Part print with two shaded views. Sizes in mm from the minimum x, y, z corner. A direction names the side the tool comes from. Round coordinates to 2 decimals unless told otherwise and drop trailing zeros. Loops run counter-clockwise (first coordinate to the right, second up) from the corner with the lowest first, then second, coordinate; pieces in that order, holes last.
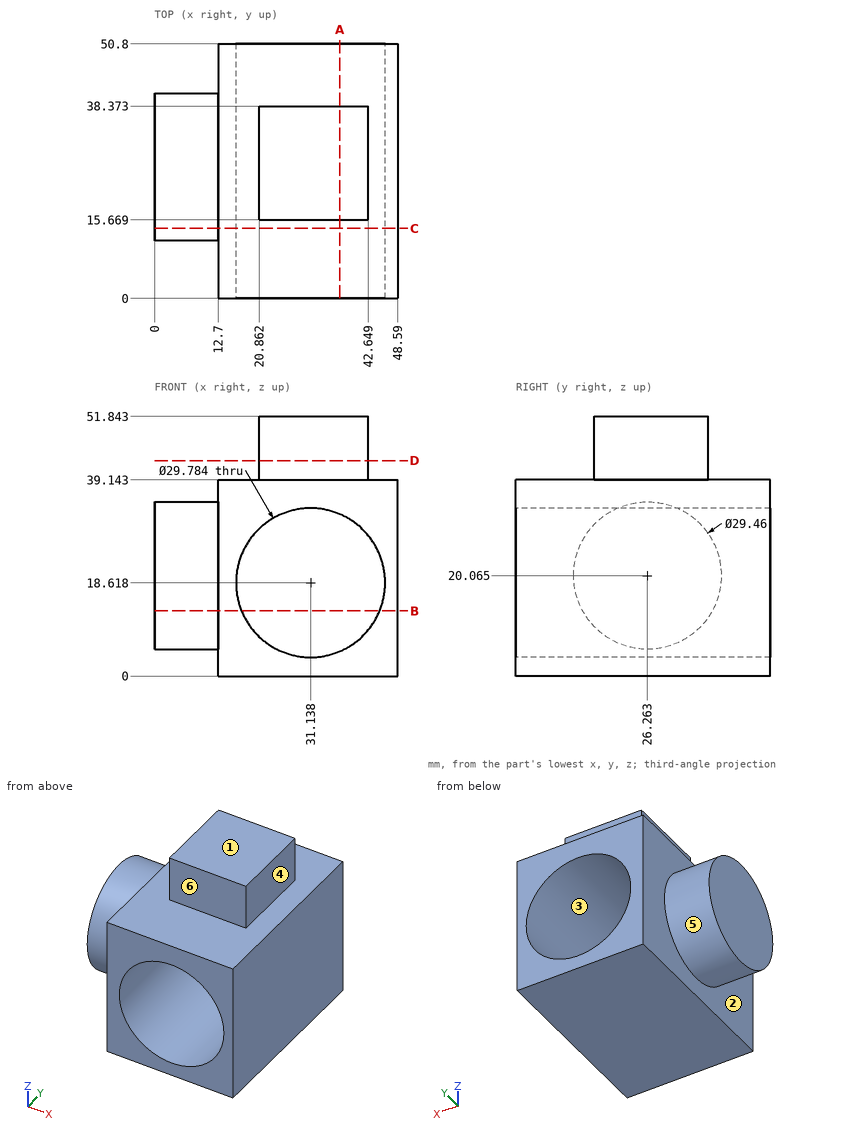
Item 1: Mould opens along X. For the marked faces 1, 2 and 3 say: released by +X, released by -X, zero draft, split by the parting line, or undercut.
Verdict:
face 1: zero draft
face 2: released by -X
face 3: undercut
Item 2: 3-axis set-ups, long thin cutter, end or side, ignore diameter. For the marked faces 4, 5 and 6: which of +Z, -Z, +X, -X, +Y, -Y reach the whole face in a straight line?
Verdict:
face 4: +Z, +X, +Y, -Y
face 5: -X
face 6: +Z, +X, -X, -Y
Item 3: Cut at C-C (y = 14). List the corners of the cut face in (x, z) (1 decimal).
Verdict:
outline: (0, 11.9) - (12.7, 11.9) - (12.7, 0) - (48.6, 0) - (48.6, 39.1) - (12.7, 39.1) - (12.7, 28.2) - (0, 28.2) - close; hole circle Ø29.8 at (31.1, 18.6)
Item 4: Cut at B-B (z = 13). List the corners of the cut face in (x, y).
Verdict:
outline: (0, 13.34) - (12.7, 13.34) - (12.7, 0) - (17.35, 0) - (17.35, 50.8) - (12.7, 50.8) - (12.7, 39.19) - (0, 39.19) - close; (44.93, 0) - (48.59, 0) - (48.59, 50.8) - (44.93, 50.8) - close
Item 5: Wall check: L1, parallel to Z at x = 30.5, y = 32.5; L2, parallel to X at y = 23, z = 38.5; L3, parallel to Z at x = 36, y = 10 (1 decimal). Give the ranges that are in metal, low to high.
Verdict:
L1: z = 0 to 3.74, 33.5 to 51.84
L2: x = 12.7 to 48.59
L3: z = 0 to 4.5, 32.7 to 39.1
Item 6: Cut at A-A (x = 37). List the corners of the cut face in (y, z).
Verdict:
outline: (0, 0) - (50.8, 0) - (50.8, 4.93) - (0, 4.93) - close; (0, 32.31) - (50.8, 32.31) - (50.8, 39.14) - (38.37, 39.14) - (38.37, 51.84) - (15.67, 51.84) - (15.67, 39.14) - (0, 39.14) - close
Item 7: Cut at D-D (z = 43). List the corners of the cut face in (x, y), plus the area to 3 significant figures.
Verdict:
outline: (20.86, 15.67) - (42.65, 15.67) - (42.65, 38.37) - (20.86, 38.37) - close
area: 495 mm2
Item 8: Flat gauge pins, fed straight in: P1, Ø6.5, axis at x = 28.5, z = 46, coming from the +Y side; P2, Ø10, axis at y = 26, z = 45, coming from the -X side; P3, Ø3, axis at x = 7, z = 26.5, coming from the +Y side. Where does each tip first touch, or does it go through?
Verdict:
P1: stops at y = 38.37
P2: stops at x = 20.86
P3: stops at y = 40.14
